```python
from build123d import *

# Parameters (mm, degrees)
SKETCH_1_W                  = 60
SKETCH_1_H                  = 131
EXTRUDE_1_DEPTH             = 5
SKETCH_2_W                  = 30
SKETCH_2_H                  = 131
EXTRUDE_2_DEPTH             = 6
SKETCH_3_R                  = 20
CUT_EXTRUDE_1_DEPTH         = 10
CHAMFER_1_SIZE              = 2
FILLET_1_R                  = 3
SKETCH_13_R                 = 1.6
CUT_EXTRUDE_2_DEPTH         = 6
SKETCH_14_R                 = 3
CUT_EXTRUDE_3_DEPTH         = 3
CHAMFER_4_SIZE              = 1
SKETCH_16_W                 = 50
SKETCH_16_H                 = 6
EXTRUDE_4_DEPTH             = 25
FILLET_3_R                  = 4
FILLET_4_R                  = 10
FILLET_5_R                  = 8
CUT_EXTRUDE_4_DEPTH         = 4
FILLET_6_R                  = 6
SKETCH_19_R                 = 2.2
CUT_EXTRUDE_5_DEPTH         = 18
SKETCH_20_R                 = 2.2
CUT_EXTRUDE_6_DEPTH         = 18
HOLE_WIZARD_M3_1_AT_2_COUNT = 2
HOLE_WIZARD_M3_1_AT_2_PITCH = 40
HOLE_WIZARD_M3_1_AT_3_COUNT = 2
HOLE_WIZARD_M3_1_AT_3_PITCH = 105.617529322
HOLE_WIZARD_M3_1_AT_4_COUNT = 2
HOLE_WIZARD_M3_1_AT_4_PITCH = 97.75
HOLE_WIZARD_M3_2_D          = 2.5
HOLE_WIZARD_M3_2_DEPTH      = 7.5
HOLE_WIZARD_M3_2_TIP        = 0.751075774


with BuildPart() as part:
    # 草图1 → 凸台-拉伸1 (new body)
    with BuildSketch(Plane.XY):
        with Locations((-207.175860782, 60.5)):
            Rectangle(SKETCH_1_W, SKETCH_1_H)
    extrude(amount=EXTRUDE_1_DEPTH)

    # 草图2 → 凸台-拉伸2 (add)
    with BuildSketch(Plane.ZY.offset(237.175860782)):
        with Locations((-10, 60.5)):
            Rectangle(SKETCH_2_W, SKETCH_2_H)
    extrude(amount=EXTRUDE_2_DEPTH)

    # 草图3 → 切除-拉伸1 (cut)
    with BuildSketch(Plane.XY.offset(5)):
        with Locations((-207.675860782, 60.5)):
            Circle(SKETCH_3_R)
    extrude(amount=-CUT_EXTRUDE_1_DEPTH, mode=Mode.SUBTRACT)

    # 倒角1
    chamfer_1_edges = [part.edges().sort_by_distance(p)[0] for p in [
        (-243.175860782, 60.5, 5),
    ]]
    chamfer(chamfer_1_edges, length=CHAMFER_1_SIZE)

    # 圆角1
    fillet_1_edges = [part.edges().sort_by_distance(p)[0] for p in [
        (-240.175860782, 126, -25),
        (-240.175860782, -5, -25),
        (-177.175860782, 126, 2.5),
        (-177.175860782, -5, 2.5),
    ]]
    fillet(fillet_1_edges, radius=FILLET_1_R)

    # 草图13 → 切除-拉伸2 (cut)
    with BuildSketch(Plane.XY.offset(5)):
        with Locations((-207.675860782, 85.5)):
            Circle(SKETCH_13_R)
        with Locations((-229.326495877, 73)):
            Circle(SKETCH_13_R)
        with Locations((-186.025225688, 73)):
            Circle(SKETCH_13_R)
        with Locations((-186.025225688, 48)):
            Circle(SKETCH_13_R)
        with Locations((-207.675860782, 35.5)):
            Circle(SKETCH_13_R)
        with Locations((-229.326495877, 48)):
            Circle(SKETCH_13_R)
    extrude(amount=-CUT_EXTRUDE_2_DEPTH, mode=Mode.SUBTRACT)

    # 草图14 → 切除-拉伸3 (cut)
    with BuildSketch(Plane.XY.offset(5)):
        with Locations((-207.675860782, 85.5)):
            Circle(SKETCH_14_R)
        with Locations((-186.025225688, 73)):
            Circle(SKETCH_14_R)
        with Locations((-186.025225688, 48)):
            Circle(SKETCH_14_R)
        with Locations((-207.675860782, 35.5)):
            Circle(SKETCH_14_R)
        with Locations((-229.326495877, 48)):
            Circle(SKETCH_14_R)
        with Locations((-229.326495877, 73)):
            Circle(SKETCH_14_R)
    extrude(amount=-CUT_EXTRUDE_3_DEPTH, mode=Mode.SUBTRACT)

    # 倒角4
    chamfer_4_edges = [part.edges().sort_by_distance(p)[0] for p in [
        (-243.175860782, 126, -9.5),
        (-242.175860782, 126, 4),
        (-210.675860782, -5, 5),
        (-242.175860782, -5, 4),
        (-243.175860782, 60.5, -25),
        (-210.675860782, 126, 5),
        (-243.175860782, -5, -9.5),
        (-243.175860782, -4.121320344, -24.121320344),
        (-243.175860782, 125.121320344, -24.121320344),
        (-177.175860782, 60.5, 5),
        (-178.054540439, -4.121320344, 5),
        (-178.054540439, 125.121320344, 5),
    ]]
    chamfer(chamfer_4_edges, length=CHAMFER_4_SIZE)

    # 草图16 → 凸台-拉伸4 (add)
    with BuildSketch(Plane(origin=(0, 0, 0), x_dir=(-1, 0, 0), z_dir=(0, 0, -1))):
        with Locations((212.175860782, 117)):
            Rectangle(SKETCH_16_W, SKETCH_16_H)
    extrude_4 = extrude(amount=EXTRUDE_4_DEPTH)

    # 镜向1: 凸台-拉伸4 across plane
    add(extrude_4.mirror(Plane(origin=(0, 60.5, 0), x_dir=(0, 0, 1), z_dir=(0, -1, 0))))

    # 圆角3
    fillet_3_edges = [part.edges().sort_by_distance(p)[0] for p in [
        (-237.175860782, -2, 0),
        (-237.175860782, 123, 0),
    ]]
    fillet(fillet_3_edges, radius=FILLET_3_R)

    # 圆角4
    fillet_4_edges = [part.edges().sort_by_distance(p)[0] for p in [
        (-237.175860782, 114, -12.5),
        (-237.175860782, 7, -12.5),
    ]]
    fillet(fillet_4_edges, radius=FILLET_4_R)

    # 圆角5
    fillet_5_edges = [part.edges().sort_by_distance(p)[0] for p in [
        (-187.175860782, 117, -25),
        (-187.175860782, 117, 0),
        (-187.175860782, 4, 0),
        (-187.175860782, 4, -25),
    ]]
    fillet(fillet_5_edges, radius=FILLET_5_R)

    # 草图17 → 切除-拉伸4 (cut)
    with BuildSketch(Plane(origin=(0, 120, 0), x_dir=(1, 0, 0), z_dir=(0, 1, 0))):
        with BuildLine():
            Line((-235.175860782, 4), (-235.175860782, 2))
            Line((-235.175860782, 2), (-233.175860782, 2))
            Line((-233.175860782, 2), (-187.175860782, 2))
            ThreePointArc((-187.175860782, 2), (-188.662693763, 4.83772234), (-189.175860782, 8))
            Line((-189.175860782, 8), (-189.175860782, 17))
            ThreePointArc((-189.175860782, 17), (-190.933220095, 21.242640687), (-195.175860782, 23))
            Line((-195.175860782, 23), (-235.175860782, 23))
            Line((-235.175860782, 23), (-235.175860782, 4))
        make_face()
    cut_extrude_4 = extrude(amount=-CUT_EXTRUDE_4_DEPTH, mode=Mode.SUBTRACT)

    # 镜向2: 切除-拉伸4 across plane
    add(cut_extrude_4.mirror(Plane(origin=(0, 60.5, 0), x_dir=(0, 0, 1), z_dir=(0, -1, 0))), mode=Mode.SUBTRACT)

    # 圆角6
    fillet_6_edges = [part.edges().sort_by_distance(p)[0] for p in [
        (-235.175860782, 118, -2),
        (-235.175860782, 118, -23),
        (-235.175860782, 3, -2),
        (-235.175860782, 3, -23),
        (-187.175860782, 118, -2),
        (-187.175860782, 3, -2),
    ]]
    fillet(fillet_6_edges, radius=FILLET_6_R - 0.0001)  # a hair under: the kernel refuses the full size

    # 草图19 → 切除-拉伸5 (cut)
    with BuildSketch(Plane.XY.offset(5)):
        with Locations((-217.175860782, -2)):
            Circle(SKETCH_19_R)
        with Locations((-187.175860782, -2)):
            Circle(SKETCH_19_R)
        with Locations((-197.175860782, -2)):
            Circle(SKETCH_19_R)
        with Locations((-207.175860782, -2)):
            Circle(SKETCH_19_R)
        with Locations((-227.175860782, -2)):
            Circle(SKETCH_19_R)
    cut_extrude_5 = extrude(amount=-CUT_EXTRUDE_5_DEPTH, mode=Mode.SUBTRACT)

    # 镜向3: 切除-拉伸5 across plane
    add(cut_extrude_5.mirror(Plane(origin=(0, 60.5, 0), x_dir=(0, 0, 1), z_dir=(0, -1, 0))), mode=Mode.SUBTRACT)

    # 草图20 → 切除-拉伸6 (cut)
    with BuildSketch(Plane.ZY.offset(243.175860782)):
        with Locations((-20.5, -2)):
            Circle(SKETCH_20_R)
        with Locations((-13, -2)):
            Circle(SKETCH_20_R)
    cut_extrude_6 = extrude(amount=-CUT_EXTRUDE_6_DEPTH, mode=Mode.SUBTRACT)

    # 镜向4: 切除-拉伸6 across plane
    add(cut_extrude_6.mirror(Plane(origin=(0, 60.5, 0), x_dir=(0, 0, 1), z_dir=(0, -1, 0))), mode=Mode.SUBTRACT)

    # 草图23 → M3 螺纹孔1 (revolve, cut)
    with BuildSketch(Plane(origin=(-229.465860782, 113.065, 5), x_dir=(0, -1, 0), z_dir=(1, 0, 0))):
        Polygon((0, 0), (0, 8.251075774), (1.25, 7.5), (1.25, 0), align=None)
    hole_wizard_m3_1 = revolve(axis=Axis((-229.465860782, 113.065, 11.35), (0, 0, -1)), mode=Mode.SUBTRACT)

    # M3 螺纹孔1 at 2: M3 螺纹孔1 ×2
    with Locations(*[(i * HOLE_WIZARD_M3_1_AT_2_PITCH, 0, 0) for i in range(1, HOLE_WIZARD_M3_1_AT_2_COUNT)]):
        add(hole_wizard_m3_1, mode=Mode.SUBTRACT)

    # M3 螺纹孔1 at 3: M3 螺纹孔1 ×2
    with Locations(*[Vector(0.3787250114344214, -0.9255092466928666, 0) * (i * HOLE_WIZARD_M3_1_AT_3_PITCH) for i in range(1, HOLE_WIZARD_M3_1_AT_3_COUNT)]):
        add(hole_wizard_m3_1, mode=Mode.SUBTRACT)

    # M3 螺纹孔1 at 4: M3 螺纹孔1 ×2
    with Locations(*[(0, -i * HOLE_WIZARD_M3_1_AT_4_PITCH, 0) for i in range(1, HOLE_WIZARD_M3_1_AT_4_COUNT)]):
        add(hole_wizard_m3_1, mode=Mode.SUBTRACT)

    # 镜向5: M3 螺纹孔1 across plane
    add(hole_wizard_m3_1.mirror(Plane(origin=(0, 60.5, 0), x_dir=(0, 0, 1), z_dir=(0, -1, 0))), mode=Mode.SUBTRACT)

    # 镜向5 copy 1 sketch → 镜向5 copy 1 (revolve, cut)
    with BuildSketch(Plane(origin=(-189.465860782, 7.935, 5), x_dir=(0, 1, 0), z_dir=(1, 0, 0))):
        Polygon((0, 0), (0, -8.251075774), (1.25, -7.5), (1.25, 0), align=None)
    revolve(axis=Axis((-189.465860782, 7.935, 11.35), (0, 0, 1)), mode=Mode.SUBTRACT)

    # 镜向5 copy 2 sketch → 镜向5 copy 2 (revolve, cut)
    with BuildSketch(Plane(origin=(-189.465860782, 105.685, 5), x_dir=(0, 1, 0), z_dir=(1, 0, 0))):
        Polygon((0, 0), (0, -8.251075774), (1.25, -7.5), (1.25, 0), align=None)
    revolve(axis=Axis((-189.465860782, 105.685, 11.35), (0, 0, 1)), mode=Mode.SUBTRACT)

    # 镜向5 copy 3 sketch → 镜向5 copy 3 (revolve, cut)
    with BuildSketch(Plane(origin=(-229.465860782, 105.685, 5), x_dir=(0, 1, 0), z_dir=(1, 0, 0))):
        Polygon((0, 0), (0, -8.251075774), (1.25, -7.5), (1.25, 0), align=None)
    revolve(axis=Axis((-229.465860782, 105.685, 11.35), (0, 0, 1)), mode=Mode.SUBTRACT)

    # M3 螺纹孔2
    with Locations(Plane.ZY.offset(243.175860782)):
        with Locations((-7.12, 85.8), (-7.12, 35.2)):
            Hole(HOLE_WIZARD_M3_2_D / 2, depth=HOLE_WIZARD_M3_2_DEPTH)
            with Locations((0, 0, -(HOLE_WIZARD_M3_2_DEPTH + HOLE_WIZARD_M3_2_TIP / 2))):  # 118° drill point
                Cone(0, HOLE_WIZARD_M3_2_D / 2, HOLE_WIZARD_M3_2_TIP, mode=Mode.SUBTRACT)


solid = part.part
```
Here's how the part is built. I have some questions about the finished solid (model axes, mm). A direction names the side the tool comes from. Round coordinates to 2 decimals unless told otherwise and drop trailing zeros. Order: outer loops, then holes, each group sorted by start corner. A loop starts at its lowest first (then second) coordinate and runs counter-clockwise, first axis right, second up. Notation, with made-up numbers: M -33.75,-16.5 L 7.25,-16.5 A28 ccw 7.25,16.5 Z; hole C 22.5,23.5 d7. An arc over 180 degrees is marked long. One line per question, with ' | ' between items.
1) For pin 1 Ø1.5 at (x, z) = (-219, -2) entering from -Y; pin 2 Ø3 at (y, z) = (24, -21) entering from +X; pin 3 Ø7 at (x, y) = (-207.68, 35.5) entering from -Z, each with a flat end and sliding along its axis, tell me the tip position at first contact or that it passes through.
Working result:
pin 1: y = 1 | pin 2: x = -237.18 | pin 3: z = 0
2) I want a section at A-A, the plane y = 48. State how many separate pieces and enclosed holes the cut face has, then the cut area to 3 significant figures.
Working result:
separate pieces: 4 | enclosed holes: 0 | area: 272 mm²
3) If we mould it in two halves opening along Y, with no side actions, what happens to faces 1 (the face through (-206.198, 84.887, 1.014)), 2 (the face through (-212, 1, -1)), 3 (the face through (-237.176, 0, -15))? For each: +Y half, -Y half, draft (parallel to the pull), parting line (faces both ways), or undercut.
Working result:
face 1: undercut | face 2: -Y half | face 3: draft
4) I need wall thicknesses on line 1 along Y through (x, z) = (-225.5, -2.5); line 2 along X through (y, z) = (60, 3); line 3 along Z through (x, y) = (-229.5, 3.5). Which ranges of each line are inside material? Lowest first, please.
Working result:
line 1: 5 to 7, 114 to 116 | line 2: -243.18 to -227.67, -187.68 to -177.18 | line 3: -25 to -22.99, -2.01 to 5
5) I want a section at B-B, the plane y = 95.5. Write out the boundary of the cut face in (x, z), then the cut area to 3 significant figures.
Working result:
outline: M -243.18,-24 L -242.18,-25 L -237.18,-25 L -237.18,0 L -177.18,0 L -177.18,4 L -178.18,5 L -241.18,5 L -243.18,3 Z | area: 477 mm²
6) For faces 4 (the face through (-212, 5, -13)), 5 (the face through (-229.521, 114.314, 2.136)), 6 (the face through (-234.324, 110.993, -12.675)), 7 (the face through (-190.98, 117.97, -3.71)), which set-ups out of +Z, -Z, +X, -X, +Y, -Y let a thin tool reach every point of the face, with its end or its side?
Working result:
face 4: -Y | face 5: +Z | face 6: -Z, +X | face 7: +Y
